```python
from build123d import *

# Parameters (mm, degrees)
CROQUIS4_R            = 3
CORTAR_EXTRUIR2_DEPTH = 10


with BuildPart() as part:
    # Croquis3 → Revolución1 (revolve)
    with BuildSketch(Plane.XY, mode=Mode.PRIVATE) as revoluci_n1_sk:
        Polygon((-18, 17.500583769), (-34, 17.500583769), (-34, -0.499416231), (-21, -0.499416231), (-21, 11.500583769), (-18, 11.500583769), align=None)
    revolve(revoluci_n1_sk.sketch.rotate(Axis((0, 0, 0), (0, 1, 0)), 270), axis=Axis((0, 0, 0), (0, 1, 0)))

    # Croquis4 → Cortar-Extruir2 (cut)
    with BuildSketch(Plane.XZ.offset(0.499416231)):
        with Locations(Location((0, 27.6, 0), (0, 0, 270))):
            Circle(CROQUIS4_R)
        with Locations(Location((27.6, 0, 0), (0, 0, 270))):
            Circle(CROQUIS4_R)
        with Locations(Location((0, -27.6, 0), (0, 0, 270))):
            Circle(CROQUIS4_R)
        with Locations(Location((-27.6, 0, 0), (0, 0, 270))):
            Circle(CROQUIS4_R)
    extrude(amount=-CORTAR_EXTRUIR2_DEPTH, mode=Mode.SUBTRACT)


solid = part.part
```
Verification items for the finished model (mm, model axes). A direction names the side the tool comes from. Give positions to 0.01 mm unless a question says otherwise; leave off trailing zeros. Loops run counter-clockwise (first coordinate to the right, second up) from the corner with the lowest first, then second, coordinate; pieces in that order, holes last.
1. Set-up check for faces 4 (the flat face through (15, 17.501, 15)), 5 (the cylindrical face through (0.9, 4.43, -30.46)): record each of +Z, -Z, +X, -X, +Y, -Y from which the full face is reachable in a straight line by a thin tool's end or side.
2. Thickness scan on line 1 (X direction, y = 3.5, z = 0); line 2 (X direction, y = 12, z = 0); line 3 (X direction, y = 4.5, z = -2.5). Record the ranges inside material, lowest first.
3. Section check C-C, the plane y = 8.5. Enter the section's corners in (x, z).
4. Section check A-A, the plane z = 0. Enter the section's corners in (x, y).
5. Section check B-B, the plane x = -8.5. Enter the section's corners in (y, z).
6. Mould release check, pull along Z, two halves, no side actions. Record for faces 1 (the cylindrical face through (-33.71, 8.37, 4.43)), 2 (the flat face through (0, 9.501, 28)), 3 (the flat face through (-16, -0.499, -15)): released by +Z, released by -Z, zero draft, split by the parting line, or undercut.
7. Section check D-D, the plane x = -25.5. Enter the section's corners in (y, z).
8. Go/stop test with flat-tipped pins: pin 1 Ø21 at (x, z) = (-10.5, 7) entering from -Y; pin 2 Ø6 at (x, y) = (-7, 13) entering from +Z; pin 3 Ø3 at (y, z) = (8.5, -9.5) entering from -X; pin 4 Ø3 at (x, z) = (26, -25) entering from +Y. Record where each tip stops, or that it passes through.
Geometry says:
1. face 4: +Z, -Z, +X, -X, +Y
1. face 5: -Y
2. line 1: x = -34 to -30.6, -24.6 to -21, 21 to 24.6, 30.6 to 34
2. line 2: x = -34 to -18, 18 to 34
2. line 3: x = -33.91 to -29.26, -25.94 to -20.85, 20.85 to 25.94, 29.26 to 33.91
3. outline: circle Ø68 at (0, 0); hole circle Ø6 at (-27.6, 0); hole circle Ø42 at (0, 0); hole circle Ø6 at (0, -27.6); hole circle Ø6 at (0, 27.6); hole circle Ø6 at (27.6, 0)
4. outline: (-34, -0.5) - (-30.6, -0.5) - (-30.6, 9.5) - (-24.6, 9.5) - (-24.6, -0.5) - (-21, -0.5) - (-21, 11.5) - (-18, 11.5) - (-18, 17.5) - (-34, 17.5) - close; (18, 11.5) - (21, 11.5) - (21, -0.5) - (24.6, -0.5) - (24.6, 9.5) - (30.6, 9.5) - (30.6, -0.5) - (34, -0.5) - (34, 17.5) - (18, 17.5) - close
5. outline: (-0.5, -32.92) - (17.5, -32.92) - (17.5, -15.87) - (11.5, -15.87) - (11.5, -19.2) - (-0.5, -19.2) - close; (-0.5, 19.2) - (11.5, 19.2) - (11.5, 15.87) - (17.5, 15.87) - (17.5, 32.92) - (-0.5, 32.92) - close
6. face 1: split by the parting line
6. face 2: undercut
6. face 3: zero draft
7. outline: (-0.5, -22.49) - (17.5, -22.49) - (17.5, 22.49) - (-0.5, 22.49) - (-0.5, 2.14) - (9.5, 2.14) - (9.5, -2.14) - (-0.5, -2.14) - close
8. pin 1: stops at y = -0.5
8. pin 2: stops at z = 33.76
8. pin 3: stops at x = -33.05
8. pin 4: passes through
